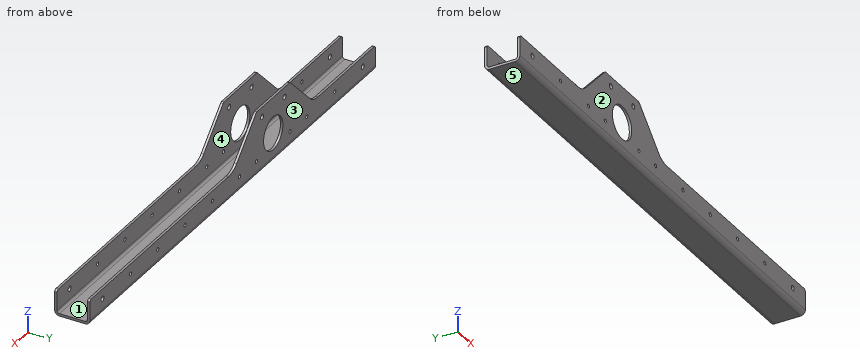
from build123d import *

# Parameters (mm, degrees)
BASE_FLANGE1_DEPTH = 647.7
SKETCH6_R          = 21.9075
CUT_EXTRUDE1_DEPTH = 655.999726679
CUT_EXTRUDE2_DEPTH = 655.999726679
SKETCH8_R          = 3.3782
SKETCH8_R_2        = 2.4257
CUT_EXTRUDE3_DEPTH = 655.999726679
SKETCH9_R          = 3.3782
CUT_EXTRUDE4_DEPTH = 655.999726679
FILLET1_R          = 25.4
FILLET2_R          = 3.175


# Sheet-metal steps are written as plain solids
with BuildPart() as part:
    # Sketch1 → Base-Flange1 (new body)
    with BuildSketch(Plane(origin=(0, 0, 0), x_dir=(0, 0, -1), z_dir=(1, 0, 0))):
        with BuildLine():
            Line((0, 0), (79.375, 0))
            ThreePointArc((79.375, 0), (81.62006403, 0.92993597), (82.55, 3.175))
            Line((82.55, 3.175), (82.55, 36.957))
            ThreePointArc((82.55, 36.957), (81.62006403, 39.20206403), (79.375, 40.132))
            Line((79.375, 40.132), (0, 40.132))
            Line((0, 40.132), (0, 43.307))
            Line((0, 43.307), (79.375, 43.307))
            ThreePointArc((79.375, 43.307), (83.865128061, 41.447128061), (85.725, 36.957))
            Line((85.725, 36.957), (85.725, 3.175))
            ThreePointArc((85.725, 3.175), (83.865128061, -1.315128061), (79.375, -3.175))
            Line((79.375, -3.175), (0, -3.175))
            Line((0, -3.175), (0, 0))
        make_face()
    extrude(amount=BASE_FLANGE1_DEPTH)

    # Sketch6 → Cut-Extrude1 (cut, through all)
    with BuildSketch(Plane(origin=(0, 43.307, 0), x_dir=(1, 0, 0), z_dir=(0, 1, 0))):
        with Locations(Location((231.775, 47.625, 0), (0, 0, 270))):
            Circle(SKETCH6_R)
    extrude(amount=-CUT_EXTRUDE1_DEPTH, mode=Mode.SUBTRACT)

    # Sketch7 → Cut-Extrude2 (cut, through all)
    with BuildSketch(Plane(origin=(0, 43.307, 0), x_dir=(1, 0, 0), z_dir=(0, 1, 0))):
        Polygon((141.2748, 52.4002), (0, 52.4002), (0, 0), (193.675, 0), align=None)
        Polygon((322.2752, 52.4002), (269.875, 0), (647.7, 0), (647.7, 52.4002), align=None)
    extrude(amount=-CUT_EXTRUDE2_DEPTH, mode=Mode.SUBTRACT)

    # Sketch8 → Cut-Extrude3 (cut, through all)
    with BuildSketch(Plane(origin=(0, 43.307, 0), x_dir=(1, 0, 0), z_dir=(0, 1, 0))):
        with Locations(Location((28.575, 65.405, 0), (0, 0, 270))):
            Circle(SKETCH8_R)
        with Locations(Location((92.075, 65.405, 0), (0, 0, 270))):
            Circle(SKETCH8_R_2)
        with Locations(Location((193.675, 65.405, 0), (0, 0, 270))):
            Circle(SKETCH8_R_2)
        with Locations(Location((269.875, 65.405, 0), (0, 0, 270))):
            Circle(SKETCH8_R_2)
        with Locations(Location((555.625, 65.405, 0), (0, 0, 270))):
            Circle(SKETCH8_R_2)
        with Locations(Location((619.125, 65.405, 0), (0, 0, 270))):
            Circle(SKETCH8_R)
        with Locations(Location((155.575, 65.405, 0), (0, 0, 270))):
            Circle(SKETCH8_R_2)
        with Locations(Location((307.975, 65.405, 0), (0, 0, 270))):
            Circle(SKETCH8_R_2)
        with Locations(Location((493.7125, 65.405, 0), (0, 0, 270))):
            Circle(SKETCH8_R_2)
        with Locations(Location((431.8, 65.405, 0), (0, 0, 270))):
            Circle(SKETCH8_R_2)
        with Locations(Location((369.8875, 65.405, 0), (0, 0, 270))):
            Circle(SKETCH8_R_2)
    extrude(amount=-CUT_EXTRUDE3_DEPTH, mode=Mode.SUBTRACT)

    # Sketch9 → Cut-Extrude4 (cut, through all)
    with BuildSketch(Plane(origin=(0, 43.307, 0), x_dir=(1, 0, 0), z_dir=(0, 1, 0))):
        with Locations(Location((257.175, 12.7, 0), (0, 0, 270))):
            Circle(SKETCH9_R)
        with Locations(Location((206.375, 12.7, 0), (0, 0, 270))):
            Circle(SKETCH9_R)
    extrude(amount=-CUT_EXTRUDE4_DEPTH, mode=Mode.SUBTRACT)

    # Fillet1
    fillet1_edges = [part.edges().sort_by_distance(p)[0] for p in [
        (141.2748, 41.7195, -52.4002),
        (141.2748, -1.5875, -52.4002),
        (322.2752, 41.7195, -52.4002),
        (322.2752, -1.5875, -52.4002),
    ]]
    fillet(fillet1_edges, radius=FILLET1_R)

    # Fillet2
    fillet2_edges = [part.edges().sort_by_distance(p)[0] for p in [
        (0, 41.7195, -52.4002),
        (193.675, 41.7195, 0),
        (193.675, -1.5875, 0),
        (0, -1.5875, -52.4002),
        (647.7, 41.7195, -52.4002),
        (269.875, 41.7195, 0),
        (647.7, -1.5875, -52.4002),
        (269.875, -1.5875, 0),
    ]]
    fillet(fillet2_edges, radius=FILLET2_R)


solid = part.part
Build history of the part. All positions in model axes, mm. Face numbers are marked on the shaded views. A direction names the side the tool comes from. Round coordinates to 2 decimals unless told otherwise and drop trailing zeros. Loops run counter-clockwise (first coordinate to the right, second up) from the corner with the lowest first, then second, coordinate; pieces in that order, holes last. Notation, with made-up numbers: (23.5, -3.5) -> (59.5, -3.5) arc R22 cw to (59.5, 23.5) -> close; hole circle Ø3 at (57.5, -3). An arc over 180 degrees is marked (long way). Use CSV: the item, a comma, the result in double quotes. Start each with the question number.
Q1. Flat gauge pins, fed straight in: pin 1 Ø1.6 at (x, y) = (414, 42.5) entering from +Z; pin 2 Ø10 at (x, y) = (363, 27.5) entering from +Z. Where does each tip first touch, or does it go through?
Q2. Saw through at A-A on x = 416.5. Give the cut face in (y, z) (3 decimals), and give its area (3 significant figures).
Q3. Mould opens along Y. For the marked faces 1, 2 and 3 say: +Y half, -Y half, draft (parallel to the pull), parting line (faces both ways), or undercut.
Q4. Saw through at B-B on y = 22.5. Give the cut face in (x, z) (3 decimals).
Q5. Drill centre lines: L1, parallel to Y at x = 320, z = -61 (3 decimals); L2, parallel to Z at x = 165, y = 8 (3 decimals); L3, parallel to X at y = 42.1, z = -12.7 (3 decimals). Where is each one in solid material? Low to high.
Q6. Which spindle directions (+Z, -Z, +X, -X, +Y, -Y) get a long thin tool onto all of the face, cutting with end or side? Do the marked faces 4 and 5. Say none if no direction does.
Solutions:
1,pin 1,"stops at z = -52.4"
1,pin 2,"stops at z = -82.55"
2,outline,"(-3.175, -79.375) arc R6.35 ccw to (3.175, -85.725) -> (36.957, -85.725) arc R6.35 ccw to (43.307, -79.375) -> (43.307, -52.4) -> (40.132, -52.4) -> (40.132, -79.375) arc R3.175 cw to (36.957, -82.55) -> (3.175, -82.55) arc R3.175 cw to (0, -79.375) -> (0, -52.4) -> (-3.175, -52.4) -> close"
2,area,"326 mm^2"
3,face 1,"undercut"
3,face 2,"-Y half"
3,face 3,"+Y half"
4,outline,"(0, -85.725) -> (647.7, -85.725) -> (647.7, -82.55) -> (0, -82.55) -> close"
5,L1,"y = -3.175 to 0, 40.132 to 43.307"
5,L2,"z = -85.725 to -82.55"
5,L3,"x = 180.975 to 202.997, 209.753 to 253.797, 260.553 to 282.575"
6,face 4,"+Z, +X, -X"
6,face 5,"-Z, +X, -X, +Y, -Y"
